```python
from build123d import *

# Parameters (mm, degrees)
CYLINDER_R                 = 3.96875
CYLINDER_DEPTH             = 50.8
EXTRUDE017_DEPTH           = 76.2
EXTRUDE017_ROLL_ANGLE      = 90
EXTRUDE017_PLACEMENT_ANGLE = 180


with BuildPart() as cylinder:
    # Cylinder → Cylinder (new body)
    with BuildSketch(Plane(origin=(381, 203.2, 16.66875), x_dir=(1, 0, 0), z_dir=(0, 0, 1))):
        Circle(CYLINDER_R)
    extrude(amount=CYLINDER_DEPTH)


with BuildPart() as baffle_anchor_a:
    # Sketch017 → Extrude017 (new body)
    with BuildSketch(Plane.XY):
        with BuildLine():
            Line((0, 41.275), (0, 3.175))
            ThreePointArc((0, 3.175), (0.929936, 0.929936), (3.175, 0))
            Line((41.275, 0), (3.175, 0))
            ThreePointArc((41.275, 0), (43.520064, 0.929936), (44.45, 3.175))
            Line((44.45, 41.275), (44.45, 3.175))
            ThreePointArc((44.45, 41.275), (43.520064, 43.520064), (41.275, 44.45))
            Line((3.175, 44.45), (41.275, 44.45))
            ThreePointArc((3.175, 44.45), (0.929936, 43.520064), (0, 41.275))
        make_face()
    extrude(amount=EXTRUDE017_DEPTH)


with BuildPart() as baffle_anchor_a_1:
    # Extrude017 roll: moved
    add(baffle_anchor_a.part.rotate(Axis((0, 0, 0), (1, 0, 0)), EXTRUDE017_ROLL_ANGLE))


with BuildPart() as baffle_anchor_a_2:
    # Extrude017 placement: moved
    add(baffle_anchor_a_1.part.moved(Location((400.05, 165.1, 19.05))).rotate(Axis((400.05, 165.1, 19.05), (0, 0, 1)), EXTRUDE017_PLACEMENT_ANGLE))

    # Cut: cut Cylinder
    add(cylinder.part, mode=Mode.SUBTRACT)


solid = baffle_anchor_a_2.part
```
Verification items for the finished model (mm, model axes). Round coordinates to 2 decimals unless told otherwise and drop trailing zeros. Order: outer loops, then holes, each group sorted by start corner. A loop starts at its lowest first (then second) coordinate and runs counter-clockwise, first axis right, second up.
1) Depth check by flat-ended pin: pin 1 (5 mm diameter, centred on x = 381, y = 203.2, fed in from -Z). Enter the tip coordinate at first touch or a pass-through.
Geometry says:
pin 1: passes through
2) Cross-section at B-B, the plane y = 203.2. Record the cut outline in (x, z) (3 decimals), plus the area to 3 significant figures.
Geometry says:
outline: (355.6, 22.225) arc R3.175 ccw to (358.775, 19.05) - (377.031, 19.05) - (377.031, 63.5) - (358.775, 63.5) arc R3.175 ccw to (355.6, 60.325) - close; (384.969, 19.05) - (396.875, 19.05) arc R3.175 ccw to (400.05, 22.225) - (400.05, 60.325) arc R3.175 ccw to (396.875, 63.5) - (384.969, 63.5) - close
area: 1,610 mm2
3) Draft check along Y on faces 1 (the flat face through (374, 203, 63.5)), 2 (the flat face through (378, 241.3, 42)), 3 (the cylindrical face through (377.035, 203.374, 40.964)). Enter one of: +Y half, -Y half, draft (parallel to the pull), parting line (faces both ways), or undercut.
Geometry says:
face 1: draft
face 2: +Y half
face 3: undercut
4) Cross-section at A-A, the plane x = 381. Record the cut outline in (y, z).
Geometry says:
outline: (165.1, 19.05) - (199.23, 19.05) - (199.23, 63.5) - (165.1, 63.5) - close; (207.17, 19.05) - (241.3, 19.05) - (241.3, 63.5) - (207.17, 63.5) - close
5) Material ranges on line 1 (X direction, y = 203.2, z = 53); line 2 (Y direction, x = 381, z = 33); line 3 (Y direction, x = 383, z = 31), recorded low to high.
Geometry says:
line 1: x = 355.6 to 377.03, 384.97 to 400.05
line 2: y = 165.1 to 199.23, 207.17 to 241.3
line 3: y = 165.1 to 199.77, 206.63 to 241.3
